Model file for the job. Use its own axes, mm. Face numbers are marked on the shaded views. A direction names the side the tool comes from. Coordinates: 2 decimals unless noted, no trailing zeros. Write each loop counter-clockwise with the first axis right and the second up, starting at its lowest first coordinate (ties: lowest second). Pieces come first, ordered by that corner, then holes. Notation, with made-up numbers: M 1,-2.75 L 30,-2.75 A11 ccw 30,17.25 Z; hole C 52.25,62.5 d5. An arc over 180 degrees is marked long. Use CSV: the item, a comma, the result in double quotes. Start each with the question number.
from build123d import *

# Parameters (mm, degrees)
F1_DEPTH = 4.7
F2_R     = 1
F3_R     = 1
F4_R     = 1
F5_R     = 1
F6_R     = 1
F7_R     = 1


with BuildPart() as f1:
    # F0 (on Top) → F1 (new body)
    with BuildSketch(Plane.XY):
        with BuildLine():
            Line((-37.863488, 16.59382), (-41.363488, 16.59382))
            add(Edge.make_bspline(
                [(-41.363488, 16.59382), (-42.3331, 8.407068), (-34.69845, 2.771639), (-27.401726, 3.610343)],
                knots=[0, 0, 0, 0, 19.065714, 19.065714, 19.065714, 19.065714], degree=3))
            Line((-27.401726, 3.610343), (-27.471585, -16.889538))
            Line((-27.471585, -16.889538), (-37.401726, -16.889538))
            Line((-37.401726, -16.889538), (-37.401726, -21.889538))
            Line((-37.401726, -21.889538), (-27.401726, -21.889538))
            Line((-27.401726, -21.889538), (-27.401726, -27.896906))
            Line((-27.401726, -27.896906), (-22.401726, -27.896906))
            Line((-22.401726, -27.896906), (-22.401726, -22.123403))
            Line((-22.401726, -22.123403), (-22.401726, 3.903857))
            add(Edge.make_bspline(
                [(-28.18239, 8.110343), (-23.64683, 7.929841), (-22.457497, 4.639071), (-22.401726, 3.903857)],
                knots=[0, 0, 0, 0, 7.149168, 7.149168, 7.149168, 7.149168], degree=3))
            add(Edge.make_bspline(
                [(-37.863488, 16.59382), (-38.216218, 11.538417), (-34.533153, 7.455524), (-28.18239, 8.110343)],
                knots=[0, 0, 0, 0, 12.87218, 12.87218, 12.87218, 12.87218], degree=3))
        make_face()
        Polygon((1.079036, -8.566779), (-22.401726, -22.123403), (-22.401726, -27.896906), (3.579036, -12.896906), align=None)
    extrude(amount=F1_DEPTH)

    # F2
    f2_edges = [f1.edges().sort_by_distance(p)[0] for p in [
        (-32.436655, -16.889538, 4.7),
        (-32.436655, -16.889538, 0),
        (-32.401726, -21.889538, 4.7),
        (-32.401726, -21.889538, 0),
    ]]
    fillet(f2_edges, radius=F2_R)

    # F3
    f3_edges = [f1.edges().sort_by_distance(p)[0] for p in [
        (-27.401726, -27.896906, 2.35),
        (-27.401726, 3.610343, 2.35),
    ]]
    fillet(f3_edges, radius=F3_R)

    # F4
    f4_edges = [f1.edges().sort_by_distance(p)[0] for p in [
        (-41.363488, 16.59382, 2.35),
        (-37.863488, 16.59382, 2.35),
    ]]
    fillet(f4_edges, radius=F4_R)

    # F5
    f5_edges = [f1.edges().sort_by_distance(p)[0] for p in [
        (-22.401726, -22.123403, 2.35),
        (1.079036, -8.566779, 2.35),
        (3.579036, -12.896906, 2.35),
        (2.329036, -10.731842, 0),
        (2.329036, -10.731842, 4.7),
    ]]
    fillet(f5_edges, radius=F5_R)

    # F6
    f6_edges = [f1.edges().sort_by_distance(p)[0] for p in [
        (-37.401726, -16.889538, 2.35),
        (-37.401726, -17.182431, 0.292893),
        (-37.401726, -17.182431, 4.407107),
        (-37.401726, -19.389538, 0),
        (-37.401726, -19.389538, 4.7),
        (-37.401726, -21.596644, 0.292893),
        (-37.401726, -21.596644, 4.407107),
        (-37.401726, -21.889538, 2.35),
    ]]
    fillet(f6_edges, radius=F6_R)

    # F7
    f7_edges = [f1.edges().sort_by_distance(p)[0] for p in [
        (-22.401726, -27.896906, 2.35),
    ]]
    fillet(f7_edges, radius=F7_R)


solid = f1.part
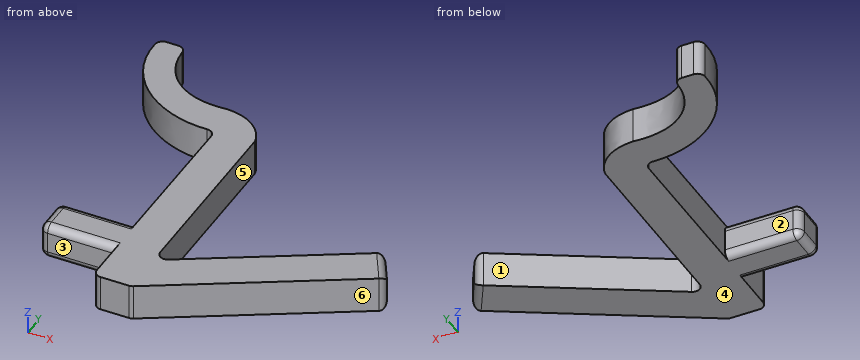
1) Tool access for the marked faces 1, 2 and 3: list every direction of +Z, -Z, +X, -X, +Y, -Y with a clear straight run to the whole face (end or side of a thin tool).
2) Band-saw the part on A-A on y = -15.5. List the corners of the cut face in (x, z).
3) Band-saw the part on B-B on x = -16. List the corners of the cut face in (y, z), then the cut area to 3 significant figures.
4) Wall check: L1, parallel to X at y = -17.5, z = 1.95; L2, parallel to X at y = -19.5, z = 3.75; L3, parallel to X at y = -0.5, z = 3.5. Give the ranges that are in metal, low to high. Write a range as [from, to].
5) Two-plate mould, pull along X, no slides. Class the marked faces 4, 5 and 6: pulls with the +X half, pulls with the -X half, needs draft (parallel to the pull), parting line crosses it, or undercut.
6) Band-saw the part on C-C on y = -7. List the corners of the cut face in (x, z).
7) Drop flat-ended pins along their axis: P1, Ø2.5, axis at y = -11, z = 3.5, coming from the +X side; P2, Ø1, axis at y = -9, z = 2.5, coming from the +X side; P3, Ø1, axis at x = -4, z = 2, coming from the -Y side. Give the stop position or say it passes through.
Findings below:
1,face 1,"+Z, -Z, +Y"
1,face 2,"+Z, -Z, -X"
1,face 3,"+Z, -Z, -X, -Y"
2,outline,"M -27.47,0 L -22.4,0 L -22.4,4.7 L -27.47,4.7 Z; M -10.93,0 L -0.93,0 L -0.93,4.7 L -10.93,4.7 Z"
3,outline,"M -24.2,0 L -18.43,0 L -18.43,4.7 L -24.2,4.7 Z"
3,area,"27.1 mm2"
4,L1,"x = [-37.32, -22.4], [-14.39, -4.39]"
4,L2,"x = [-37.4, -22.4], [-17.86, -7.86]"
4,L3,"x = [-27.42, -22.4]"
5,face 4,"needs draft"
5,face 5,"undercut"
5,face 6,"pulls with the +X half"
6,outline,"M -27.44,0 L -22.4,0 L -22.4,4.7 L -27.44,4.7 Z"
7,P1,"stops at x = 3.17"
7,P2,"stops at x = 1.62"
7,P3,"stops at y = -17.56"
